Could you check a few things on this drawing? It's one solid part, dimensions in mm from its lowest x, y, z. Give positions to 0.01 mm unless a question says otherwise; leave off trailing zeros. Loops run counter-clockwise (first coordinate to the right, second up) from the corner with the lowest first, then second, coordinate; pieces in that order, holes last. Notation, with made-up numbers: (-28.5, -9) - (-19.5, -9) arc R32 ccw to (-19.5, 25) - close; hole circle Ø6 at (-4.75, 76.5). An arc over 180 degrees is marked (long way). Return JSON: item names as keys, results as strings. Group by question number.
(1) If we section it at B-B (z = 11.95): Please give me the cut outline in (x, y), then the cut area to 3 significant figures.
(2) If we section it at D-D (y = 0.5): Please give me the cut outline in (x, z), then the cut area to 3 significant figures.
(3) If we section it at C-C (y = 3): Please give me the cut outline in (x, z), then the cut area to 3 significant figures.
(4) For P1, Ø2, axis at x = 5.5, y = 5.5, coming from the -Z side; P2, Ø1.5, axis at y = 6, z = 8.5, coming from the +X side; P3, Ø5, axis at x = 3.5, y = 4.5, coming from the -Z side; P4, Ø6, axis at x = 11.95, z = 11.95, coming from the +Y side, each with a flat end and sliding along its axis, tell me the tip position at first contact or that it passes through.
(5) I need wall thicknesses on probe 1 along Z at (x, y) = (12, 7.5); probe 2 along Z at (x, y) = (11.5, 9.5). Which ranges of each line are inside material? Lowest first, please. Write a range as [from, to].
(6) If we section it at A-A (x = 11.95): Please give me the cut outline in (y, z).
(7) If we mould it in two halves opening along Z, with no side actions, what happens to the marked faces 1, 2 and 3? For each: released by +Z, released by -Z, zero draft, split by the parting line, or undercut.
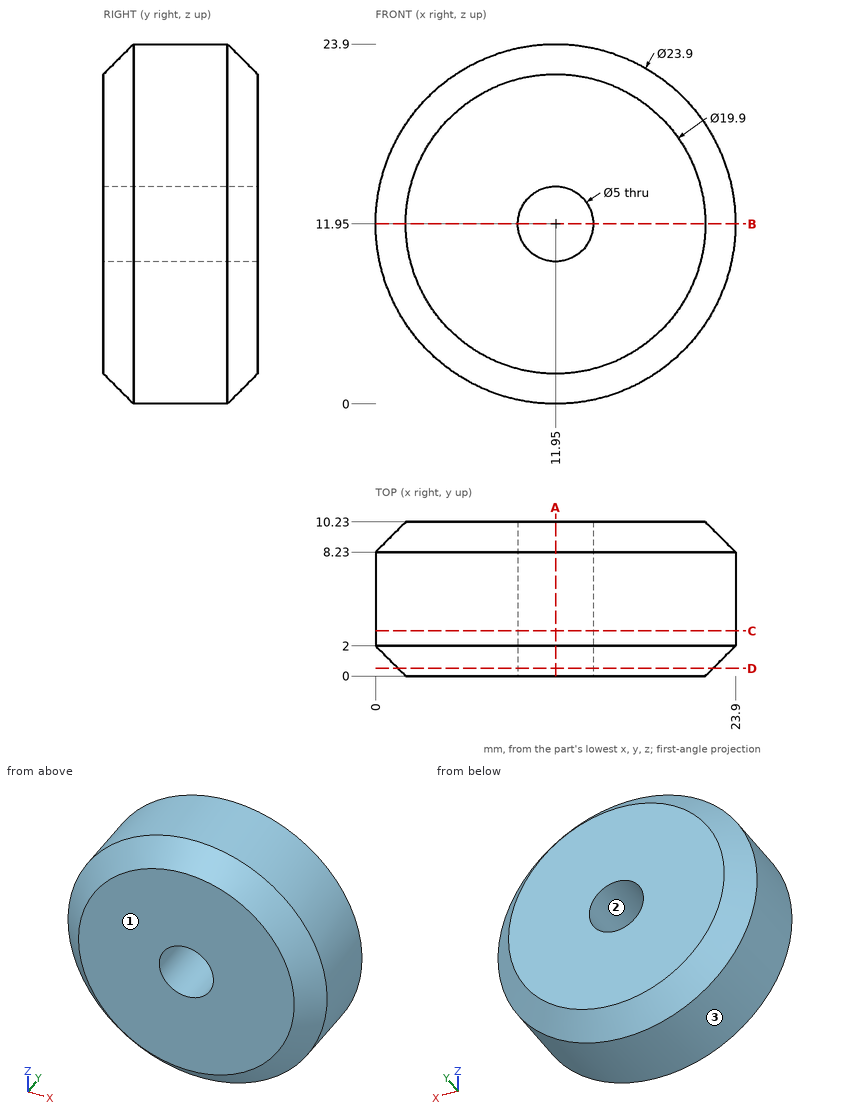
Values:
{
 "1": {"outline": "(0, 2) - (2, 0) - (9.45, 0) - (9.45, 10.23) - (2, 10.23) - (0, 8.23) - close; (14.45, 0) - (21.9, 0) - (23.9, 2) - (23.9, 8.23) - (21.9, 10.23) - (14.45, 10.23) - close", "area": "185 mm2"},
 "2": {"outline": "circle Ø20.9 at (11.95, 11.95); hole circle Ø5 at (11.95, 11.95)", "area": "323 mm2"},
 "3": {"outline": "circle Ø23.9 at (11.95, 11.95); hole circle Ø5 at (11.95, 11.95)", "area": "429 mm2"},
 "4": {"P1": "z = 1.32", "P2": "x = 23.59", "P3": "z = 1.59", "P4": "y = 10.23"},
 "5": {"probe 1": "[0, 9.45], [14.45, 23.9]", "probe 2": "[1.28, 9.49], [14.41, 22.62]"},
 "6": {"outline": "(0, 2) - (2, 0) - (8.23, 0) - (10.23, 2) - (10.23, 9.45) - (0, 9.45) - close; (0, 14.45) - (10.23, 14.45) - (10.23, 21.9) - (8.23, 23.9) - (2, 23.9) - (0, 21.9) - close"},
 "7": {"face 1": "zero draft", "face 2": "undercut", "face 3": "split by the parting line"}
}
